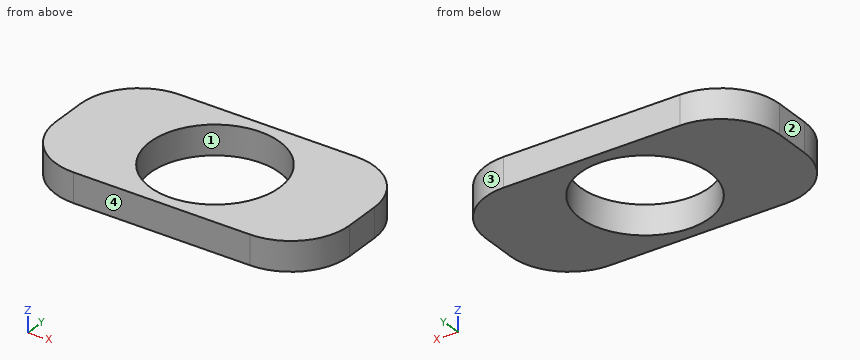
from build123d import *

# Parameters (mm, degrees)
F0_R     = 11.025
F1_DEPTH = 2.5
F4_R     = 10


with BuildPart() as f1:
    # F0 (on Top) → F1 (new body, symmetric)
    with BuildSketch(Plane.XY):
        with BuildLine():
            ThreePointArc((0, -13.025), (-13.025, 0), (0, 13.025))
            Line((0, 13.025), (-25, 13.025))
            Line((-25, 13.025), (-25, -13.025))
            Line((-25, -13.025), (0, -13.025))
        make_face()
        with BuildLine():
            ThreePointArc((0, 13.025), (9.210066, 9.210066), (13.025, 0))
            ThreePointArc((13.025, 0), (9.210066, -9.210066), (0, -13.025))
            Line((0, -13.025), (25, -13.025))
            Line((25, -13.025), (25, 13.025))
            Line((25, 13.025), (0, 13.025))
        make_face()
        with BuildLine():
            ThreePointArc((0, -13.025), (9.210066, -9.210066), (13.025, 0))
            ThreePointArc((13.025, 0), (9.210066, 9.210066), (0, 13.025))
            ThreePointArc((0, 13.025), (-13.025, 0), (0, -13.025))
        make_face()
        Circle(F0_R, mode=Mode.SUBTRACT)
    extrude(amount=F1_DEPTH, both=True)

    # F2 (on Right) → F3 (revolve, cut)
    with BuildSketch(Plane.YZ):
        with BuildLine():
            Line((6.4, 2.5), (5.430738, 2.5))
            Line((5.430738, 2.5), (5.430738, -2.5))
            Line((5.430738, -2.5), (6.4, -2.5))
            add(Edge.make_bspline(
                [(6.4, 2.5), (6.199995, 1.666646), (6.3, -2.1e-05), (6.200005, -1.666687), (6.4, -2.5)],
                knots=[0, 0, 0, 0, 2.504557, 5.008992, 5.008992, 5.008992, 5.008992], degree=3))
        make_face()
    revolve(axis=Axis((0, 0, 5.107941), (0, 0, 1)), mode=Mode.SUBTRACT)

    # F4
    f4_edges = [f1.edges().sort_by_distance(p)[0] for p in [
        (-25, -13.025, 0),
        (-25, 13.025, 0),
        (25, -13.025, 0),
        (25, 13.025, 0),
    ]]
    fillet(f4_edges, radius=F4_R)


solid = f1.part
Can you work these out from the model? Positions are in its coordinate system, mm. Face numbers are marked on the shaded views. Give positions to 0.01 mm unless a question says otherwise; leave off trailing zeros. Order: outer loops, then holes, each group sorted by start corner. A loop starts at its lowest first (then second) coordinate and runs counter-clockwise, first axis right, second up. Notation, with made-up numbers: M -23,52.25 L -4,52.25 A30 ccw -4,76.25 Z; hole C 0,35.25 d1. An arc over 180 degrees is marked long. Use a Markdown table: item, result. Add a question column.
Item 1: Will this pin go through, and if not, where does the flat tip stop? pin 1 (1.5 mm diameter, centred on x = 17, z = 0, fed in from +Y).
Item 2: Suppose I cut it at B-B (x = 0). List the corners of the cut face in (y, z) for me (3 decimals).
Item 3: Suppose I cut it at D-D (x = -21.5). List the corners of the cut face in (y, z) for me, then the cut area to 3 significant figures.
Item 4: We'd pull the mould along Y, two halves only. Please class the marked faces 1, 2, 3 and 4: +Y half, -Y half, draft (parallel to the pull), parting line (faces both ways), or undercut.
Item 5: Suppose I cut it at C-C (y = 0). List the corners of the cut face in (x, z) for me (3 decimals).
Item 6: If I drill on L1, parallel to Y at x = 0, z = 0.3 (3 decimals); L2, parallel to X at y = 2.75, z = 0.2; L3, parallel to X at y = 5, z = -1.4, over which ranges is the centre line in solid material (lowest first)? Write a range as [from, to].
Item 7: Suppose I cut it at A-A (z = -0.65). List the corners of the cut face in (x, y) for me (3 decimals), then the cut area to 3 significant figures.
Answer sheet:
| question | item | result |
|---|---|---|
| 1 | pin 1 | stops at y = 12.95 |
| 2 | outline | M -13.025,-2.5 L -11.025,-2.5 L -11.025,2.5 L -13.025,2.5 Z; M 11.025,-2.5 L 13.025,-2.5 L 13.025,2.5 L 11.025,2.5 Z |
| 3 | outline | M -10.62,-2.5 L 10.62,-2.5 L 10.62,2.5 L -10.62,2.5 Z |
| 3 | area | 106 mm² |
| 4 | face 1 | undercut |
| 4 | face 2 | draft |
| 4 | face 3 | +Y half |
| 4 | face 4 | -Y half |
| 5 | outline | M -25,-2.5 L -11.025,-2.5 L -11.025,2.5 L -25,2.5 Z; M 11.025,-2.5 L 25,-2.5 L 25,2.5 L 11.025,2.5 Z |
| 6 | L1 | y = [-13.025, -11.025], [11.025, 13.025] |
| 6 | L2 | x = [-25, -10.68], [10.68, 25] |
| 6 | L3 | x = [-24.8, -9.83], [9.83, 24.8] |
| 7 | outline | M -25,-3.025 A10 ccw -15,-13.025 L 15,-13.025 A10 ccw 25,-3.025 L 25,3.025 A10 ccw 15,13.025 L -15,13.025 A10 ccw -25,3.025 Z; hole C 0,0 d22.05 |
| 7 | area | 835 mm² |
